Here's how the part is built. I have some questions about the finished solid (model axes, mm). A direction names the side the tool comes from. Give positions to 0.01 mm unless a question says otherwise; leave off trailing zeros. Loops run counter-clockwise (first coordinate to the right, second up) from the corner with the lowest first, then second, coordinate; pieces in that order, holes last. Notation, with made-up numbers: M -8.75,-33.5 L 20.25,-33.5 A19 ccw 20.25,-2.5 Z; hole C -27,69.5 d5. An arc over 180 degrees is marked long. Answer as CSV lines item,"result". Start each with the question number.
Item 1: I want a section at A-A on z = 1. List the corners of the cut face in (x, y) for me, plus the area to 3 significant figures.
Item 2: I want a section at D-D on z = 8. List the corners of the cut face in (x, y) for me.
Item 3: I want a section at C-C on x = 5. List the corners of the cut face in (y, z) for me, plus the area to 3 significant figures.
Item 4: I want a section at B-B on y = 20. List the corners of the cut face in (x, z) for me, plus the area to 3 significant figures.
Item 5: If we mould it in two halves opening along X, with no side actions, what happens to faces 4 (the flat face through (-6.15, 4.47, 4.93)), 5 (the flat face through (-9.8, 16, 4.9)), 6 (the flat face through (-21.752, -12.325, 4.93)), 7 (the flat face through (6, 2, 0))? For each: released by +X, released by -X, zero draft, split by the parting line, or undercut.
Item 6: If I drill on line 1 along Y through (x, z) = (-6.5, 3.25); line 2 along Y through (x, z) = (-12.5, 2); line 3 along Y through (x, z) = (-7, 4.5), over which ranges is the centre line in solid material (lowest first)? Write a range as from..to.
Item 7: For faces 1 (the flat face through (9.85, 15.85, 4.93)), 2 (the flat face through (0, -5, 10)), 3 (the flat face through (0, -11, 3)), which set-ups out of +Z, -Z, +X, -X, +Y, -Y let a thin tool reach every point of the face, with its end or its side?
Item 8: Will these pins go through, and if not, where does the flat tip stop? P1, Ø4, axis at y = 16, z = 8, coming from the -X side; P2, Ø3, axis at y = -18, z = 7.5, coming from the -X side; P3, Ø5, axis at y = -11.5, z = 3.5, coming from the -X side; P4, Ø1, axis at y = -4, z = 3.5, coming from the +X side.
from build123d import *

# Parameters (mm, degrees)
SKETCH001_W           = 80
SKETCH001_H           = 8
EXTRUDE001_DEPTH      = 5
EXTRUDE001_DEPTH_BACK = 1
SKETCH_W              = 20
SKETCH_H              = 4
EXTRUDE_DEPTH         = 10


with BuildPart() as extrude001:
    # Sketch001 → Extrude001 (new body, two sides)
    with BuildSketch(Plane.XY) as extrude001_sk:
        with Locations((0, -7)):
            Rectangle(SKETCH001_W, SKETCH001_H)
    extrude(amount=EXTRUDE001_DEPTH)
    extrude(extrude001_sk.sketch, amount=-EXTRUDE001_DEPTH_BACK)


with BuildPart() as cut:
    # Sketch → Extrude (new body)
    with BuildSketch(Plane.XY):
        Polygon((28.867513, 0), (14.433757, 25), (-14.433757, 25), (-28.867513, 0), (-14.433757, -25), (14.433757, -25), align=None)
        Polygon((7.5, 23.082627), (-7.5, 23.082627), (-12.135255, 8.816779), (0, 0), (12.135255, 8.816779), align=None, mode=Mode.SUBTRACT)
        with Locations((0, -17)):
            Rectangle(SKETCH_W, SKETCH_H, mode=Mode.SUBTRACT)
    extrude(amount=EXTRUDE_DEPTH)

    # Cut: cut Extrude001
    add(extrude001.part, mode=Mode.SUBTRACT)


solid = cut.part
Result:
1,outline,"M -28.87,0 L -27.14,-3 L 27.14,-3 L 28.87,0 L 14.43,25 L -14.43,25 Z; M -22.52,-11 L -14.43,-25 L 14.43,-25 L 22.52,-11 Z; hole M -12.14,8.82 L 0,0 L 12.14,8.82 L 7.5,23.08 L -7.5,23.08 Z; hole M -10,-19 L 10,-19 L 10,-15 L -10,-15 Z"
1,area,"1,300 mm^2"
2,outline,"M -28.87,0 L -14.43,-25 L 14.43,-25 L 28.87,0 L 14.43,25 L -14.43,25 Z; hole M -12.14,8.82 L 0,0 L 12.14,8.82 L 7.5,23.08 L -7.5,23.08 Z; hole M -10,-19 L 10,-19 L 10,-15 L -10,-15 Z"
3,outline,"M -25,0 L -19,0 L -19,10 L -25,10 Z; M -15,0 L -11,0 L -11,5 L -3,5 L -3,0 L 3.63,0 L 3.63,10 L -15,10 Z; M 23.08,0 L 25,0 L 25,10 L 23.08,10 Z"
3,area,"226 mm^2"
4,outline,"M -17.32,0 L -8.5,0 L -8.5,10 L -17.32,10 Z; M 8.5,0 L 17.32,0 L 17.32,10 L 8.5,10 Z"
4,area,"176 mm^2"
5,face 4,"undercut"
5,face 5,"undercut"
5,face 6,"released by -X"
5,face 7,"zero draft"
6,line 1,"-25..-19, -15..-11, -3..4.72, 23.08..25"
6,line 2,"-25..-11, -3..25"
6,line 3,"-25..-19, -15..-11, -3..5.09, 23.08..25"
7,face 1,"+Z, -Z"
7,face 2,"+Z, +X, -X, +Y, -Y"
7,face 3,"-Z, +X, -X"
8,P1,"x = -20.78"
8,P2,"x = -19.34"
8,P3,"x = -23.38"
8,P4,"through"
